from build123d import *

# Parameters (mm, degrees)
F0_W     = 76.2
F0_H     = 50.8
F0_W_2   = 50.8
F0_H_2   = 25.4
F1_DEPTH = 63.5
F2_R     = 19.05
F3_W     = 38.1
F3_H     = 63.5
F4_DEPTH = 127


with BuildPart() as f1:
    # F0 (on Front) → F1 (new body)
    with BuildSketch(Plane.XZ):
        Rectangle(F0_W, F0_H)
        with Locations((0.819354, -0.819356)):
            Rectangle(F0_W_2, F0_H_2, mode=Mode.SUBTRACT)
    extrude(amount=F1_DEPTH)

    # F2
    f2_edges = [f1.edges().sort_by_distance(p)[0] for p in [
        (38.1, -31.75, 25.4),
        (38.1, -31.75, -25.4),
    ]]
    fillet(f2_edges, radius=F2_R)

    # F3 (on Front) → F4 (join)
    with BuildSketch(Plane.XZ):
        with Locations((-57.149999, -1.467527)):
            Rectangle(F3_W, F3_H)
    extrude(amount=F4_DEPTH)


solid = f1.part
Verification items for the finished model (mm, model axes). A direction names the side the tool comes from. Coordinates: 2 decimals unless noted, no trailing zeros. Loops run counter-clockwise (first coordinate to the right, second up) from the corner with the lowest first, then second, coordinate; pieces in that order, holes last. Notation, with made-up numbers: (62, 44.25) -> (75, 44.25) arc R28 ccw to (75, 82.25) -> close; hole circle Ø4 at (-19, -10). An arc over 180 degrees is marked (long way). Answer as a JSON object with one key per item and string values. Group by question number.
Item 1: Depth check by flat-ended pin: pin 1 (15 mm diameter, centred on x = 4, y = -24.5, fed in from +Z); pin 2 (1 mm diameter, centred on x = 7.5, z = 14, fed in from -Y); pin 3 (12 mm diameter, centred on y = -35, z = 13, fed in from +X). Enter the tip coordinate at first touch or a pass-through.
Item 2: Sectioned sample at A-A on x = 17. Record the boundary of the cut face in (y, z).
Item 3: Sectioned sample at D-D on y = -72. Record the boundary of the cut face in (x, z).
Item 4: Sectioned sample at B-B on z = -8.5. Record the boundary of the cut face in (x, y).
Item 5: Tool access check on faces 1 (the flat face through (-10, -31, -25.4)), 2 (the flat face through (-1, -63.5, 17)), 3 (the flat face through (26.219, -31, -1)), 4 (the flat face through (-10, -31, 25.4)). Record the directions out of +Z, -Z, +X, -X, +Y, -Y that give a thin tool (end or side, any length) a straight path to the whole face; none if there is none.
Item 6: Scan lines: probe 1 along Z at (x, y) = (-15.5, -5.5); probe 2 along X at (y, z) = (-54, 2); probe 3 along X at (y, z) = (-68.5, 13). Record each from-to range of solid material in increasing order.
Item 7: Mould release check, pull along X, two halves, no side actions. Record for faces 5 (the flat face through (-33, 0, -1)), 6 (the flat face through (-76.2, -63, -2)), 7 (the flat face through (-24.581, -31, -1)): +X half, -X half, draft (parallel to the pull), parting line (faces both ways), or undercut.
Item 8: Sectioned sample at C-C on y = -44. Record the boundary of the cut face in (x, z).
Evaluation:
{
 "1": {"pin 1": "stops at z = 25.4", "pin 2": "stops at y = -63.5", "pin 3": "stops at x = 38.09"},
 "2": {"outline": "(-63.5, -25.4) -> (0, -25.4) -> (0, -13.52) -> (-63.5, -13.52) -> close; (-63.5, 11.88) -> (0, 11.88) -> (0, 25.4) -> (-63.5, 25.4) -> close"},
 "3": {"outline": "(-76.2, -33.22) -> (-38.1, -33.22) -> (-38.1, 30.28) -> (-76.2, 30.28) -> close"},
 "4": {"outline": "(-76.2, -127) -> (-38.1, -127) -> (-38.1, -63.5) -> (-24.58, -63.5) -> (-24.58, 0) -> (-76.2, 0) -> close; (26.22, -63.5) -> (37.98, -63.5) -> (37.98, 0) -> (26.22, 0) -> close"},
 "5": {"face 1": "-Z, +X, +Y, -Y", "face 2": "+Z, -Z, +X, -Y", "face 3": "+Y, -Y", "face 4": "+Z, +X, +Y, -Y"},
 "6": {"probe 1": "z = -25.4 to -13.52, 11.88 to 25.4", "probe 2": "x = -76.2 to -24.58, 26.22 to 38.1", "probe 3": "x = -76.2 to -38.1"},
 "7": {"face 5": "draft", "face 6": "-X half", "face 7": "undercut"},
 "8": {"outline": "(-76.2, -33.22) -> (-38.1, -33.22) -> (-38.1, -25.4) -> (19.05, -25.4) arc R19.05 ccw to (38.1, -6.35) -> (38.1, 6.35) arc R19.05 ccw to (19.05, 25.4) -> (-38.1, 25.4) -> (-38.1, 30.28) -> (-76.2, 30.28) -> close; hole (-24.58, -13.52) -> (26.22, -13.52) -> (26.22, 11.88) -> (-24.58, 11.88) -> close"}
}
